The model under review builds one solid part; all positions refer to its coordinate system, in mm. A direction names the side the tool comes from. Coordinates: 2 decimals unless noted, no trailing zeros. Write each loop counter-clockwise with the first axis right and the second up, starting at its lowest first coordinate (ties: lowest second). Pieces come first, ordered by that corner, then holes. Notation, with made-up numbers: (72.25, 60.25) - (123.25, 60.25) arc R22 cw to (123.25, 89.25) - close; hole circle Ø2 at (25.25, 65). An arc over 180 degrees is marked (long way). Return JSON: item names as keys, results as strings. Group by question number.
(1) We need section B-B on x = 20.32. State the section outline as (y, z) points (3 decimals).
(2) Tool access review of faces 1 (the face through (-16.51, 2, 6)), 2 (the face through (22, 3.81, 3)), 3 (the face through (-7, 3.81, 5)): name each direction out of +Z, -Z, +X, -X, +Y, -Y from which nothing blocks a thin tool from reaching the whole face with its end or side.
(3) We need section D-D on x = 5.08. State the section outline as (y, z) points.
(4) We need section A-A on z = 6.35. State the section outline as (x, y) points (3 decimals).
(5) Draft analysis for pull direction X (two halves, no side actions). For faces 4 (the face through (5.24, 9.67, 6.26)), 5 (the face through (17.15, 1.93, 6.21)), 6 (the face through (4.97, 5.08, 6.26)), 7 (the face through (-6.5, 0, 6.3)), state which applies: released by +X, released by -X, zero draft, split by the parting line, or undercut.
(6) We need section C-C on z = 2. State the section outline as (x, y) points, then the cut area to 3 significant figures.
(7) For pin 1 Ø2 at (y, z) = (8.5, 7) entering from +X; pin 2 Ø2 at (y, z) = (5, 3) entering from -X, all flat-tipped, find the tip position at first contact; note any pin that passes through.
(8) To check wall thickness, follow L1, parallel to Z at x = 20.32, y = 1.4 (3 decimals); L2, parallel to Y at x = -11, z = 2.5; L3, parallel to X at y = 2.75, z = 11.75. State the ranges of each line that lie inside material, in increasing order. Write a range as from..to.
```python
from build123d import *

# Parameters (mm, degrees)
BOSS_EXTRUDE1_DEPTH = 12.7
SKETCH2_R           = 3.175
CUT_EXTRUDE1_DEPTH  = 31.115483017


with BuildPart() as part:
    # Sketch1 → Boss-Extrude1 (new body)
    with BuildSketch(Plane.XY):
        with BuildLine():
            Line((-3.81, 3.81), (-16.51, 3.81))
            Line((-16.51, 3.81), (-16.51, 0))
            Line((-16.51, 0), (0, 0))
            ThreePointArc((0, 0), (5.08, 5.08), (10.16, 0))
            Line((10.16, 0), (26.67, 0))
            Line((26.67, 0), (26.67, 3.81))
            Line((26.67, 3.81), (13.97, 3.81))
            ThreePointArc((13.97, 3.81), (5.08, 9.672031844), (-3.81, 3.81))
        make_face()
    extrude(amount=BOSS_EXTRUDE1_DEPTH)

    # Sketch2 → Cut-Extrude1 (cut, through all)
    with BuildSketch(Plane(origin=(0, 3.81, 0), x_dir=(1, 0, 0), z_dir=(0, 1, 0))):
        with Locations(Location((-10.16, -6.35, 0), (0, 0, 180))):
            Circle(SKETCH2_R)
        with Locations((20.32, -6.35)):
            Circle(SKETCH2_R)
    extrude(amount=-CUT_EXTRUDE1_DEPTH, mode=Mode.SUBTRACT)


solid = part.part
```
Ans:
{
 "1": {"outline": "(0, 0) - (3.81, 0) - (3.81, 3.175) - (0, 3.175) - close; (0, 9.525) - (3.81, 9.525) - (3.81, 12.7) - (0, 12.7) - close"},
 "2": {"face 1": "+Z, -Z, -X, +Y, -Y", "face 2": "+Z, -Z, +X, +Y", "face 3": "+Z, -Z, -X, +Y"},
 "3": {"outline": "(5.08, 0) - (9.67, 0) - (9.67, 12.7) - (5.08, 12.7) - close"},
 "4": {"outline": "(-16.51, 0) - (-13.335, 0) - (-13.335, 3.81) - (-16.51, 3.81) - close; (-6.985, 0) - (0, 0) arc R5.08 cw to (10.16, 0) - (17.145, 0) - (17.145, 3.81) - (13.97, 3.81) arc R9.672 ccw to (-3.81, 3.81) - (-6.985, 3.81) - close; (23.495, 0) - (26.67, 0) - (26.67, 3.81) - (23.495, 3.81) - close"},
 "5": {"face 4": "split by the parting line", "face 5": "undercut", "face 6": "undercut", "face 7": "zero draft"},
 "6": {"outline": "(-16.51, 0) - (0, 0) arc R5.08 cw to (10.16, 0) - (26.67, 0) - (26.67, 3.81) - (13.97, 3.81) arc R9.67 ccw to (-3.81, 3.81) - (-16.51, 3.81) - close", "area": "199 mm²"},
 "7": {"pin 1": "x = 11.19", "pin 2": "x = -3.73"},
 "8": {"L1": "0..3.175, 9.525..12.7", "L2": "0..3.81", "L3": "-16.51..0.81, 9.35..26.67"}
}
